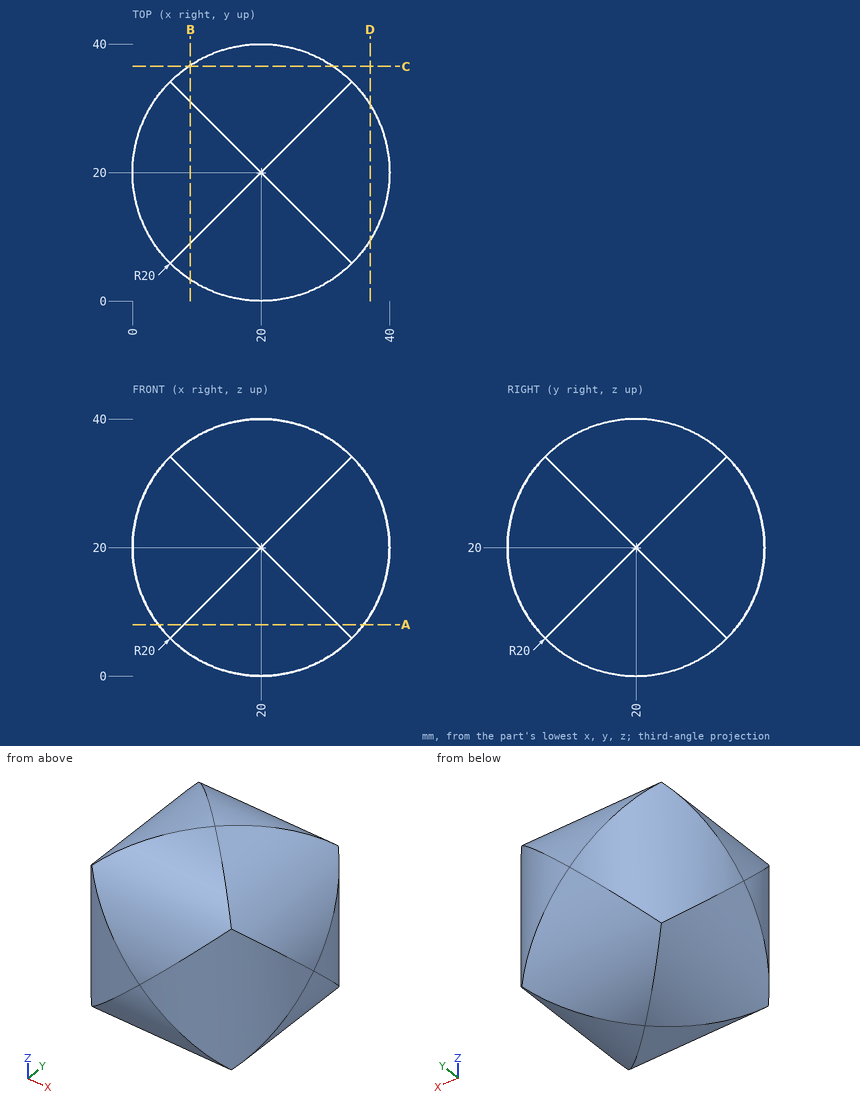
Drawing for the job (mm, zero at the part's lowest x, y, z). Give positions to 0.01 mm unless a question says otherwise; leave off trailing zeros. Loops run counter-clockwise (first coordinate to the right, second up) from the corner with the lowest first, then second, coordinate; pieces in that order, holes last.
(1) Band-saw the part on A-A (z = 8). Write the cut outline in (x, y), and give its area (3 significant figures).
Return value:
outline: (4, 8) arc R20 ccw to (8, 4) - (32, 4) arc R20 ccw to (36, 8) - (36, 32) arc R20 ccw to (32, 36) - (8, 36) arc R20 ccw to (4, 32) - close
area: 995 mm2
(2) Pin check, flat tips, straight feed: pin 1 (5 mm diameter, centred on y = 27.5, z = 28, fed in from +X); pin 2 (5 mm diameter, centred on x = 30.5, y = 7, fed in from +Z); pin 3 (8 mm diameter, centred on x = 8.5, z = 36, fed in from +Y). Stop position of each tip, or through.
Return value:
pin 1: stops at x = 39.08
pin 2: stops at z = 37.02
pin 3: stops at y = 36
(3) Drill centre lines: line 1 along Y through (x, z) = (27.5, 22); line 2 along Z through (x, y) = (4, 28.5); line 3 along Z through (x, y) = (14, 37). Where is each one in solid material? Low to high.
Return value:
line 1: y = 1.46 to 38.54
line 2: z = 8 to 32
line 3: z = 9.46 to 30.54
(4) Band-saw the part on D-D (x = 37). Write the cut outline in (y, z).
Return value:
outline: (9.46, 9.46) - (30.54, 9.46) - (30.54, 30.54) - (9.46, 30.54) - close
(5) Band-saw the part on B-B (x = 9). Write the cut outline in (y, z), and give its area (3 significant figures).
Return value:
outline: (3.3, 9) arc R20 ccw to (9, 3.3) - (31, 3.3) arc R20 ccw to (36.7, 9) - (36.7, 31) arc R20 ccw to (31, 36.7) - (9, 36.7) arc R20 ccw to (3.3, 31) - close
area: 1,060 mm2
(6) Band-saw the part on C-C (y = 36.5). Write the cut outline in (x, z), and give its area (3 significant figures).
Return value:
outline: (8.7, 8.7) - (31.3, 8.7) - (31.3, 31.3) - (8.7, 31.3) - close
area: 511 mm2
